```python
from build123d import *

# Parameters (mm, degrees)
SKETCH1_R           = 1.5
SKETCH1_W           = 3
SKETCH1_H           = 10
SKETCH1_W_2         = 10
SKETCH1_H_2         = 3
BOSS_EXTRUDE1_DEPTH = 3


with BuildPart() as part:
    # Sketch1 → Boss-Extrude1 (new body)
    with BuildSketch(Plane.XY):
        Polygon((-54.478363627, 39.675247502), (-54.478363627, 36.675247502), (-34.478363627, 36.675247502), (-34.478363627, 39.675247502), (35.521636373, 39.675247502), (35.521636373, 36.675247502), (55.521636373, 36.675247502), (55.521636373, 39.675247502), (65.521636373, 39.675247502), (65.521636373, -40.324752498), (55.521636373, -40.324752498), (55.521636373, -37.324752498), (35.521636373, -37.324752498), (35.521636373, -40.324752498), (-34.478363627, -40.324752498), (-34.478363627, -37.324752498), (-54.478363627, -37.324752498), (-54.478363627, -40.324752498), (-64.478363627, -40.324752498), (-64.478363627, 39.675247502), align=None)
        with Locations((16.34767445, 14.599209425)):
            Circle(SKETCH1_R, mode=Mode.SUBTRACT)
        with Locations((-14.65232555, 14.599209425)):
            Circle(SKETCH1_R, mode=Mode.SUBTRACT)
        with Locations((16.34767445, -16.400790575)):
            Circle(SKETCH1_R, mode=Mode.SUBTRACT)
        with Locations((-14.65232555, -16.400790575)):
            Circle(SKETCH1_R, mode=Mode.SUBTRACT)
        with Locations((22.5, 0)):
            Rectangle(SKETCH1_W, SKETCH1_H, mode=Mode.SUBTRACT)
        with Locations((-21.978363627, -0.324752498)):
            Rectangle(SKETCH1_W, SKETCH1_H, mode=Mode.SUBTRACT)
        with BuildLine():
            Line((-60.228363627, 10.675247502), (-34.228363627, 10.675247502))
            ThreePointArc((-34.228363627, 10.675247502), (-32.228363627, 8.675247502), (-34.228363627, 6.675247502))
            Line((-34.228363627, 6.675247502), (-60.228363627, 6.675247502))
            ThreePointArc((-60.228363627, 6.675247502), (-62.228363627, 8.675247502), (-60.228363627, 10.675247502))
        make_face(mode=Mode.SUBTRACT)
        with BuildLine():
            Line((-34.228363627, -7.324752498), (-60.228363627, -7.324752498))
            ThreePointArc((-60.228363627, -7.324752498), (-62.228363627, -9.324752498), (-60.228363627, -11.324752498))
            Line((-60.228363627, -11.324752498), (-34.228363627, -11.324752498))
            ThreePointArc((-34.228363627, -11.324752498), (-32.228363627, -9.324752498), (-34.228363627, -7.324752498))
        make_face(mode=Mode.SUBTRACT)
        with BuildLine():
            Line((35.271636373, 10.675247502), (61.271636373, 10.675247502))
            ThreePointArc((61.271636373, 10.675247502), (63.271636373, 8.675247502), (61.271636373, 6.675247502))
            Line((61.271636373, 6.675247502), (35.271636373, 6.675247502))
            ThreePointArc((35.271636373, 6.675247502), (33.271636373, 8.675247502), (35.271636373, 10.675247502))
        make_face(mode=Mode.SUBTRACT)
        with BuildLine():
            Line((35.271636373, -7.324752498), (61.271636373, -7.324752498))
            ThreePointArc((61.271636373, -7.324752498), (63.271636373, -9.324752498), (61.271636373, -11.324752498))
            Line((61.271636373, -11.324752498), (35.271636373, -11.324752498))
            ThreePointArc((35.271636373, -11.324752498), (33.271636373, -9.324752498), (35.271636373, -7.324752498))
        make_face(mode=Mode.SUBTRACT)
        with Locations((33.427979094, -16.824752498)):
            Rectangle(SKETCH1_W_2, SKETCH1_H_2, mode=Mode.SUBTRACT)
        with Locations((33.427979094, 16.175247502)):
            Rectangle(SKETCH1_W_2, SKETCH1_H_2, mode=Mode.SUBTRACT)
        with Locations((0.521636373, -3.574752498)):
            Rectangle(SKETCH1_W_2, SKETCH1_H_2, mode=Mode.SUBTRACT)
        with Locations((0.521636373, 2.925247502)):
            Rectangle(SKETCH1_W_2, SKETCH1_H_2, mode=Mode.SUBTRACT)
    extrude(amount=BOSS_EXTRUDE1_DEPTH)


solid = part.part
```
Can you work these out from the model? Positions are in its coordinate system, mm. A direction names the side the tool comes from. Coordinates: 2 decimals unless noted, no trailing zeros. Loops run counter-clockwise (first coordinate to the right, second up) from the corner with the lowest first, then second, coordinate; pieces in that order, holes last.
1) For pin 1 (0.9 mm diameter, centred on x = 45, z = 1, fed in from -Y); pin 2 (1 mm diameter, centred on x = -37, z = 1.5, fed in from +Y), each with a flat end and sliding along its axis, tell me the tip position at first contact or that it passes through.
2) Which directions (+Z, -Z, +X, -X, +Y, -Y) give clear straight access to the entire face, cutting with the end or side of a thin tool? Please do faces 4 (the flat face through (-34.478, 38, 1)), 5 (the flat face through (-47, 10.675, 1)), 6 (the flat face through (35.522, -39, 1)).
3) I need wall thicknesses on probe 1 along X at (y, z) = (4.5, 0.5); probe 2 along Y at (x, z) = (-54, 0.2); probe 3 along X at (y, z) = (-4, 0.9). Which ranges of each line are inside material? Lowest first, please.
4) Imagine slicing it at B-B on x = 47. List the corners of the cut face in (y, z) for me, plus the area to 3 significant figures.
5) Imagine slicing it at C-C on z = 2.1. State how many separate pieces and enclosed holes the cut face has, plus the area to 3 significant figures.
6) Thinking about a two-plate mould opening in Y: for faces 1 (the flat face through (45, 36.675, 1)), 2 (the flat face through (24, 0, 1)), 3 (the flat face through (61, -40.325, 1)), which applies, pulls with the +Y half, pulls with the -Y half, needs draft (parallel to the pull), parting line crosses it, or undercut?
7) Imagine slicing it at A-A on x = 30. List the corners of the cut face in (y, z) for me, plus the area to 3 significant figures.
Completed:
1. pin 1: stops at y = -37.32
1. pin 2: stops at y = 36.68
2. face 4: +Z, -Z, +Y
2. face 5: +Z, -Z
2. face 6: +Z, -Z, -Y
3. probe 1: x = -64.48 to -23.48, -20.48 to 21, 24 to 65.52
3. probe 2: y = -37.32 to -11.32, -7.32 to 6.68, 10.68 to 36.68
3. probe 3: x = -64.48 to -23.48, -20.48 to -4.48, 5.52 to 21, 24 to 65.52
4. outline: (-37.32, 0) - (-11.32, 0) - (-11.32, 3) - (-37.32, 3) - close; (-7.32, 0) - (6.68, 0) - (6.68, 3) - (-7.32, 3) - close; (10.68, 0) - (36.68, 0) - (36.68, 3) - (10.68, 3) - close
4. area: 198 mm2
5. separate pieces: 1
5. enclosed holes: 14
5. area: 9,490 mm2
6. face 1: pulls with the +Y half
6. face 2: undercut
6. face 3: pulls with the -Y half
7. outline: (-40.32, 0) - (-18.32, 0) - (-18.32, 3) - (-40.32, 3) - close; (-15.32, 0) - (14.68, 0) - (14.68, 3) - (-15.32, 3) - close; (17.68, 0) - (39.68, 0) - (39.68, 3) - (17.68, 3) - close
7. area: 222 mm2
